Design review of the part built by this model. Coordinates are the model's own, in mm. A direction names the side the tool comes from. Give positions to 0.01 mm unless a question says otherwise; leave off trailing zeros. Loops run counter-clockwise (first coordinate to the right, second up) from the corner with the lowest first, then second, coordinate; pieces in that order, holes last. Notation, with made-up numbers: (59.5, -17) -> (70.5, -17) arc R18 ccw to (70.5, -4) -> close; hole circle Ø6 at (79.25, -10). An arc over 180 degrees is marked (long way). Use a Markdown table: item, result. Add a question column.
1. Add section A-A (z = 10). State the section outline as (x, y) points.
2. For pin 1 Ø8 at (x, z) = (271.5, 1.5) entering from -Y; pin 2 Ø8 at (y, z) = (387, 11.5) entering from +X; pin 3 Ø5 at (y, z) = (451, 13) entering from -X; pin 4 Ø8 at (y, z) = (562, 8) entering from -X, all flat-tipped, find the tip position at first contact; note any pin that passes through.
3. Add section C-C (x = 62). State the section outline as (y, z) points.
4. To check wall thickness, follow line 1 (Y direction, x = 564, z = 1); line 2 (X direction, y = 483, z = 14.75); line 3 (Y direction, x = 263.5, z = 15). State the ranges of each line that lie inside material, in increasing order.
5. For faces 1 (the flat face through (624, 477.5, 8)), 2 (the flat face through (207, 510, 8)), 3 (the flat face through (690, 505, 8)), 4 (the flat face through (690, 555, 8)), list the 3-axis set-ups (+Z, -Z, +X, -X, +Y, -Y) from which the entire face can be reached by the end or side of a thin tool; tool diameter is ignored.
6. Draft analysis for pull direction Y (two halves, no side actions). For faces 5 (the flat face through (570, 138, 8)), 6 (the flat face through (548, 580, 8)), 7 (the flat face through (680, 390, 8)), state which applies: pulls with the +Y half, pulls with the -Y half, needs draft (parallel to the pull), parting line crosses it, or undercut.
7. Add section B-B (y = 521.5). State the section outline as (x, z) points, and give its area (3 significant figures).
```python
from build123d import *

# Parameters (mm, degrees)
SKETCH1_W           = 680
SKETCH1_H           = 560
BOSS_EXTRUDE1_DEPTH = 16
SKETCH2_W           = 550
SKETCH2_H           = 20
BOSS_EXTRUDE2_DEPTH = 16
SKETCH3_W           = 70
SKETCH3_H           = 80
CUT_EXTRUDE1_DEPTH  = 17
CUT_EXTRUDE2_REACH  = 18
SKETCH4_W           = 570
SKETCH4_H           = 320
SKETCH4_H_2         = 70
SKETCH5_W           = 20
SKETCH5_H           = 50
SKETCH5_H_2         = 70
SKETCH5_H_3         = 370
BOSS_EXTRUDE3_DEPTH = 16
SKETCH6_W           = 150
SKETCH6_H           = 70
BOSS_EXTRUDE4_DEPTH = 16


with BuildPart() as part:
    # Sketch1 → Boss-Extrude1 (new body)
    with BuildSketch(Plane.XY):
        with Locations((340, 280)):
            Rectangle(SKETCH1_W, SKETCH1_H)
    extrude(amount=BOSS_EXTRUDE1_DEPTH)

    # Sketch2 → Boss-Extrude2 (add)
    with BuildSketch(Plane.XY.offset(16)):
        with Locations((405, -10)):
            Rectangle(SKETCH2_W, SKETCH2_H)
        with Locations((405, 570)):
            Rectangle(SKETCH2_W, SKETCH2_H)
    extrude(amount=-BOSS_EXTRUDE2_DEPTH)

    # Sketch3 → Cut-Extrude1 (cut, through all)
    with BuildSketch(Plane.XY.offset(16)):
        with Locations((624, 437.5)):
            Rectangle(SKETCH3_W, SKETCH3_H)
    extrude(amount=-CUT_EXTRUDE1_DEPTH, mode=Mode.SUBTRACT)

    # Sketch4 → Cut-Extrude2 (cut, up to next)
    with BuildSketch(Plane.XY.offset(16), mode=Mode.PRIVATE) as cut_extrude2_sk1:
        with Locations((285, 140)):
            Rectangle(SKETCH4_W, SKETCH4_H)
    cut_extrude2_tool1 = extrude(cut_extrude2_sk1.sketch, amount=-CUT_EXTRUDE2_REACH, mode=Mode.PRIVATE) & part.part
    add(cut_extrude2_tool1.solids().sort_by_distance((285, 140, 16))[0], mode=Mode.SUBTRACT)
    # Sketch4 → Cut-Extrude2 (cut, up to next)
    with BuildSketch(Plane.XY.offset(16), mode=Mode.PRIVATE) as cut_extrude2_sk2:
        with Locations((285, 545)):
            Rectangle(SKETCH4_W, SKETCH4_H_2)
    cut_extrude2_tool2 = extrude(cut_extrude2_sk2.sketch, amount=-CUT_EXTRUDE2_REACH, mode=Mode.PRIVATE) & part.part
    add(cut_extrude2_tool2.solids().sort_by_distance((285, 545, 16))[0], mode=Mode.SUBTRACT)

    # Sketch5 → Boss-Extrude3 (add)
    with BuildSketch(Plane.XY.offset(16)):
        with Locations((690, 530)):
            Rectangle(SKETCH5_W, SKETCH5_H)
        with Locations((690, 440)):
            Rectangle(SKETCH5_W, SKETCH5_H_2)
        with Locations((690, 190)):
            Rectangle(SKETCH5_W, SKETCH5_H_3)
    extrude(amount=-BOSS_EXTRUDE3_DEPTH)

    # Sketch6 → Boss-Extrude4 (add)
    with BuildSketch(Plane.XY.offset(16)):
        with Locations((495, 545)):
            Rectangle(SKETCH6_W, SKETCH6_H)
    extrude(amount=-BOSS_EXTRUDE4_DEPTH)


solid = part.part
```
Taken from the geometry:
| question | item | result |
|---|---|---|
| 1 | outline | (0, 300) -> (570, 300) -> (570, -20) -> (680, -20) -> (680, 5) -> (700, 5) -> (700, 375) -> (680, 375) -> (680, 405) -> (700, 405) -> (700, 475) -> (680, 475) -> (680, 505) -> (700, 505) -> (700, 555) -> (680, 555) -> (680, 580) -> (420, 580) -> (420, 510) -> (0, 510) -> close; hole (589, 397.5) -> (659, 397.5) -> (659, 477.5) -> (589, 477.5) -> close |
| 2 | pin 1 | stops at y = 300 |
| 2 | pin 2 | stops at x = 680 |
| 2 | pin 3 | stops at x = 0 |
| 2 | pin 4 | stops at x = 420 |
| 3 | outline | (300, 0) -> (510, 0) -> (510, 16) -> (300, 16) -> close |
| 4 | line 1 | y = 300 to 580 |
| 4 | line 2 | x = 0 to 680 |
| 4 | line 3 | y = 300 to 510 |
| 5 | face 1 | +Z, -Z |
| 5 | face 2 | +Z, -Z, -X, +Y |
| 5 | face 3 | +Z, -Z, +X |
| 5 | face 4 | +Z, -Z, +X, +Y |
| 6 | face 5 | needs draft |
| 6 | face 6 | pulls with the +Y half |
| 6 | face 7 | undercut |
| 7 | outline | (420, 0) -> (700, 0) -> (700, 16) -> (420, 16) -> close |
| 7 | area | 4,480 mm^2 |
